Geometry check sheet. Reference: the model listing, model coordinates, mm. A direction names the side the tool comes from. Give positions to 0.01 mm unless a question says otherwise; leave off trailing zeros. Order: outer loops, then holes, each group sorted by start corner. A loop starts at its lowest first (then second) coordinate and runs counter-clockwise, first axis right, second up. Notation, with made-up numbers: M 6,37.5 L 49,37.5 A18 cw 49,70.5 Z; hole C 87.25,31.25 d3. An arc over 180 degrees is marked long. Use CSV: the item, a comma, the result in double quotes. Start each with the question number.
from build123d import *

# Parameters (mm, degrees)
AUFSATZ_AUFTRAGEN_MAIN_BODY_DEPTH = 40
SKIZZE3_R                         = 8.75
BOHRUNG_HORIZONTAL_DEPTH          = 115.821600755
SKIZZE4_R                         = 8.75
BOHRUNG_VERTIKAL_DEPTH            = 115.821600755


with BuildPart() as part:
    # Skizze1 → Aufsatz Auftragen Main Body (new, symmetric)
    with BuildSketch(Plane.XY):
        with BuildLine():
            Line((0, 0), (80, 0))
            Line((80, 0), (80, 8))
            Line((80, 8), (18, 8))
            ThreePointArc((18, 8), (10.928932188, 10.928932188), (8, 18))
            Line((8, 18), (8, 80))
            Line((8, 80), (0, 80))
            Line((0, 80), (0, 0))
        make_face()
    extrude(amount=AUFSATZ_AUFTRAGEN_MAIN_BODY_DEPTH, both=True)

    # Skizze3 → Bohrung Horizontal (cut, through all)
    with BuildSketch(Plane(origin=(0, 8, 0), x_dir=(1, 0, 0), z_dir=(0, 1, 0))):
        with Locations(Location((45, 0, 0), (0, 0, 180))):
            Circle(SKIZZE3_R)
    extrude(amount=-BOHRUNG_HORIZONTAL_DEPTH, mode=Mode.SUBTRACT)

    # Skizze4 → Bohrung Vertikal (cut, through all)
    with BuildSketch(Plane(origin=(8, 0, 0), x_dir=(0, 0, -1), z_dir=(1, 0, 0))):
        with Locations(Location((0, 45, 0), (0, 0, 90))):
            Circle(SKIZZE4_R)
    extrude(amount=-BOHRUNG_VERTIKAL_DEPTH, mode=Mode.SUBTRACT)


solid = part.part
(1) Access from +Z, -Z, +X, -X, +Y, -Y to the whole of each face (thin tool, end or side, straight path). Record for faces 5 (the face through (8, 55, 1)), 6 (the face through (4, 80, 1)).
(2) Sectioned sample at B-B on y = 45. Record the cut outline in (x, z).
(3) Thickness scan on line 1 (Z direction, x = 45, y = 2.5); line 2 (X direction, y = 31.5, z = 35). Record the ranges inside material, lowest first.
(4) Sectioned sample at D-D on z = -17.5. Record the cut outline in (x, y).
(5) Go/stop test with flat-tipped pins: P1, Ø23, axis at y = 45, z = 0, coming from the +X side; P2, Ø1, axis at y = 13.5, z = 1, coming from the +X side; P3, Ø5, axis at x = 65, z = 21, coming from the +Y side; P4, Ø4, axis at x = 46, z = -5.5, coming from the -Y side. Record where each tip stops, or that it passes through.
(6) Sectioned sample at A-A on z = 0. Record the cut outline in (x, y), then the cut area to 3 significant figures.
(7) Draft check along Z on faces 1 (the face through (7, 22, -40)), 2 (the face through (46.9, 4.06, -8.54)), 3 (the face through (11.01, 10.85, 0.56)), 4 (the face through (7, 22, 40)). Enter one of: +Z half, -Z half, draft (parallel to the pull), parting line (faces both ways), or undercut.
Responses:
1,face 5,"+Z, -Z, +X, +Y"
1,face 6,"+Z, -Z, +X, -X, +Y"
2,outline,"M 0,-40 L 8,-40 L 8,-8.75 L 0,-8.75 Z; M 0,8.75 L 8,8.75 L 8,40 L 0,40 Z"
3,line 1,"-40 to -8.75, 8.75 to 40"
3,line 2,"0 to 8"
4,outline,"M 0,0 L 80,0 L 80,8 L 18,8 A10 cw 8,18 L 8,80 L 0,80 Z"
5,P1,"x = 8"
5,P2,"x = 9.34"
5,P3,"y = 8"
5,P4,"through"
6,outline,"M 0,0 L 36.25,0 L 36.25,8 L 18,8 A10 cw 8,18 L 8,36.25 L 0,36.25 Z; M 0,53.75 L 8,53.75 L 8,80 L 0,80 Z; M 53.75,0 L 80,0 L 80,8 L 53.75,8 Z"
6,area,"957 mm2"
7,face 1,"-Z half"
7,face 2,"undercut"
7,face 3,"draft"
7,face 4,"+Z half"
